Here's how the part is built. I have some questions about the finished solid (model axes, mm). A direction names the side the tool comes from. Coordinates: 2 decimals unless noted, no trailing zeros. Loops run counter-clockwise (first coordinate to the right, second up) from the corner with the lowest first, then second, coordinate; pieces in that order, holes last.
from build123d import *

# Parameters (mm, degrees)
F0_W     = 43.18
F0_H     = 5.08
F1_DEPTH = 19.05
F3_DEPTH = 58.42
F4_R     = 5.08
F5_R     = 2.413
F6_DEPTH = 25.4


with BuildPart() as f1:
    # F0 (on Front) → F1 (new body, symmetric)
    with BuildSketch(Plane.XZ):
        with Locations((0, -13.789871)):
            Rectangle(F0_W, F0_H)
    extrude(amount=F1_DEPTH, both=True)

    # F2 (on face) → F3 (join)
    with BuildSketch(Plane.XY.offset(-11.249871)):
        Polygon((10.448596, 6.0325), (0, 12.065), (-10.448596, 6.0325), (-10.448596, -6.0325), (0, -12.065), (10.448596, -6.0325), align=None)
        Polygon((-8.248892, 4.7625), (0, 9.525), (8.248892, 4.7625), (8.248892, -4.7625), (0, -9.525), (-8.248892, -4.7625), align=None, mode=Mode.SUBTRACT)
    extrude(amount=F3_DEPTH)

    # F4
    f4_edges = [f1.edges().sort_by_distance(p)[0] for p in [
        (10.448596, 0, -11.249871),
        (5.224298, -9.04875, -11.249871),
        (-5.224298, -9.04875, -11.249871),
        (5.224298, 9.04875, -11.249871),
        (-5.224298, 9.04875, -11.249871),
        (-10.448596, 0, -11.249871),
    ]]
    fillet(f4_edges, radius=F4_R)

    # F5 (on face) → F6 (cut)
    with BuildSketch(Plane(origin=(0, 0, -16.329871), x_dir=(1, 0, 0), z_dir=(0, 0, -1))):
        with Locations((-14.351, 11.557)):
            Circle(F5_R)
        with Locations((14.351, 11.557)):
            Circle(F5_R)
        with Locations((-14.351, -11.557)):
            Circle(F5_R)
        with Locations((14.351, -11.557)):
            Circle(F5_R)
    extrude(amount=-F6_DEPTH, mode=Mode.SUBTRACT)


solid = f1.part
Q1. Suppose I cut it at A-A on z = 41. Write out the boundary of the cut face in (x, y) (1 decimal), and give its area (3 significant figures).
Q2. Will these pins go through, and if not, where does the flat tip stop? P1, Ø5.5, axis at x = 14.351, y = -11.557, coming from the -Z side; P2, Ø4, axis at y = -11, z = 26, coming from the -X side; P3, Ø7.5, axis at y = -1, z = 7.5, coming from the +X side; P4, Ø3, axis at y = 8.5, z = 37, coming from the -X side.
Q3. For faces 4 (the flat face through (4.2, -7.1, 17.6)), 5 (the flat face through (-5.297, -9.007, 20.127)), 6 (the flat face through (-5.15, 9.09, 20.13)), which set-ups out of +Z, -Z, +X, -X, +Y, -Y let a thin tool reach every point of the face, with its end or its side?
Q4. We'd pull the mould along Y, two halves only. Please class faces 1 (the flat face through (5.297, 9.007, 20.127)), 2 (the flat face through (-10, -13, -11.25)), 3 (the cylindrical face through (11.94, 11.45, -13.8)): pulls with the +Y half, pulls with the -Y half, needs draft (parallel to the pull), parting line crosses it, or undercut.
Q5. Suppose I cut it at B-B on y = -1. Write out the boundary of the cut face in (x, z).
Q6. Please list where these lines run through material, in increasing order: probe 1 along X at (y, z) = (-2, 45); probe 2 along Z at (x, y) = (-7, 14); probe 3 along Y at (x, z) = (0, -4) (3 decimals).
Check values:
1. outline: (-10.4, -6) - (0, -12.1) - (10.4, -6) - (10.4, 6) - (0, 12.1) - (-10.4, 6) - close; hole (-8.2, -4.8) - (0, -9.5) - (8.2, -4.8) - (8.2, 4.8) - (0, 9.5) - (-8.2, 4.8) - close
1. area: 142 mm2
2. P1: stops at z = -16.33
2. P2: stops at x = -5.31
2. P3: stops at x = 10.45
2. P4: stops at x = -8.77
3. face 4: +Z
3. face 5: +Z, -X, -Y
3. face 6: +Z, -X, +Y
4. face 1: pulls with the +Y half
4. face 2: needs draft
4. face 3: undercut
5. outline: (-21.59, -16.33) - (21.59, -16.33) - (21.59, -11.25) - (15.53, -11.25) arc R5.08 cw to (10.45, -6.17) - (10.45, 47.17) - (8.25, 47.17) - (8.25, -11.25) - (-8.25, -11.25) - (-8.25, 47.17) - (-10.45, 47.17) - (-10.45, -6.17) arc R5.08 cw to (-15.53, -11.25) - (-21.59, -11.25) - close
6. probe 1: x = -10.45 to -8.25, 8.25 to 10.45
6. probe 2: z = -16.33 to -11.25
6. probe 3: y = -12.065 to -9.525, 9.525 to 12.065
